from build123d import *

# Parameters (mm, degrees)
F1_DEPTH       = 25.4
F2_SIZE        = 20.32
F5_R           = 6.35
F6_DEPTH       = 25.4
F6_DEPTH_BACK  = 25.4
F7_R           = 3.81
F8_DEPTH       = 46.228
F8_DEPTH_BACK  = 55.88
F9_R           = 6.35
F10_DEPTH      = 25.4
F10_DEPTH_BACK = 25.4
F11_R          = 3.81
F12_DEPTH      = 41.402
F12_DEPTH_BACK = 45.212
F13_R          = 5.08


# Not quite as in the source:
# - a feature of the source that left no trace in its solid (it failed there, or was rolled back) is left out


with BuildPart() as f1:
    # F0 (on Front) → F1 (new body)
    with BuildSketch(Plane.XZ):
        Polygon((0, 57.15), (-25.0849546432, 41.8481773181), (-25.0849546432, -41.8481773181), (0, -57.15), (25.0849546432, -41.8481773181), (25.0849546432, 41.8481773181), align=None)
    extrude(amount=F1_DEPTH)

    # F2
    f2_edges = [f1.edges().sort_by_distance(p)[0] for p in [
        (-12.542477, -25.4, 49.499089),
        (12.542477, -25.4, 49.499089),
    ]]
    chamfer(f2_edges, length=F2_SIZE)

    # F5 (on Right) → F6 (join, two sides)
    with BuildSketch(Plane.YZ) as f6_sk:
        with Locations((0, -29.1547831148)):
            Circle(F5_R)
    extrude(amount=-F6_DEPTH)
    extrude(f6_sk.sketch, amount=F6_DEPTH_BACK)

    # F7 (on Right) → F8 (cut, two sides)
    with BuildSketch(Plane.YZ) as f8_sk:
        with Locations((0, -29.1547831148)):
            Circle(F7_R)
    extrude(amount=-F8_DEPTH, mode=Mode.SUBTRACT)
    extrude(f8_sk.sketch, amount=F8_DEPTH_BACK, mode=Mode.SUBTRACT)

    # F9 (on Right) → F10 (join, two sides)
    with BuildSketch(Plane.YZ) as f10_sk:
        with Locations((0, 22.8599980474)):
            Circle(F9_R)
    extrude(amount=F10_DEPTH)
    extrude(f10_sk.sketch, amount=-F10_DEPTH_BACK)

    # F11 (on Right) → F12 (cut, two sides)
    with BuildSketch(Plane.YZ) as f12_sk:
        with Locations((0, 22.8599980474)):
            Circle(F11_R)
    extrude(amount=-F12_DEPTH, mode=Mode.SUBTRACT)
    extrude(f12_sk.sketch, amount=F12_DEPTH_BACK, mode=Mode.SUBTRACT)

    # F13
    f13_edges = [f1.edges().sort_by_distance(p)[0] for p in [
        (-25.084955, -25.4, -11.901086),
        (-12.542477, -25.4, 25.696917),
        (-12.542477, -25.4, -49.499089),
        (12.542477, -25.4, 25.696917),
        (12.542477, -25.4, -49.499089),
        (25.084955, -25.4, -11.901086),
    ]]
    fillet(f13_edges, radius=F13_R)


solid = f1.part
The model under review builds one solid part; all positions refer to its coordinate system, in mm. A direction names the side the tool comes from. Give positions to 0.01 mm unless a question says otherwise; leave off trailing zeros. Write each loop counter-clockwise with the first axis right and the second up, starting at its lowest first coordinate (ties: lowest second). Pieces come first, ordered by that corner, then holes. Notation, with made-up numbers: M -28.5,86.25 L -10.5,86.25 A19 ccw -10.5,94.25 Z; hole C 49.5,-8.75 d3. An arc over 180 degrees is marked long. One line per question, with ' | ' between items. Start each with the question number.
Item 1: For pin 1 (4.5 mm diameter, centred on y = 0, z = 22.86, fed in from +X); pin 2 (19.5 mm diameter, centred on x = 10.5, z = -2, fed in from +Y); pin 3 (6 mm diameter, centred on y = -12, z = 6.5, fed in from +X); pin 4 (1 mm diameter, centred on y = -15.5, z = -19.5, fed in from -X), all flat-tipped, find the tip position at first contact; note any pin that passes through.
Item 2: For faces 1 (the flat face through (0, 0, 40)), 2 (the flat face through (0, 0, -44)), 3 (the flat face through (25.085, -10, -1)), list the 3-axis set-ups (+Z, -Z, +X, -X, +Y, -Y) from which the entire face can be reached by the end or side of a thin tool; tool diameter is ignored.
Item 3: We need section A-A on z = -26.5. Write out the cut boundary in (x, y), plus the area to 3 significant figures.
Item 4: We need section B-B on y = -14. Write out the cut boundary in (x, z), plus the area to 3 significant figures.
Item 5: We need section C-C on z = 14.5. Write out the cut boundary in (x, y).
Item 6: We need section D-D on x = 3.5. Give the number of separate pieces and of enclosed holes in the cut face, plus the area to 3 significant figures.
Item 7: Wall thickness on line 1 (Z direction, x = -3, y = 0.5); line 2 (Y direction, x = -1.5, z = 14.5); line 3 (X direction, y = -10.5, z = -19): over which ranges is each line inside the solid? List them lowest first. Write a range as from..to.
Results found:
1) pin 1: passes through | pin 2: stops at y = 0 | pin 3: stops at x = 25.08 | pin 4: stops at x = -25.08
2) face 1: +Z, +X, -X, +Y | face 2: -Z, +X, -X, +Y | face 3: +X, -Y
3) outline: M -25.4,-5.77 L -25.08,-5.77 L -25.08,-20.32 A5.08 ccw -20,-25.4 L 20,-25.4 A5.08 ccw 25.08,-20.32 L 25.08,-5.77 L 25.4,-5.77 L 25.4,-2.73 L -25.4,-2.73 Z; M -25.4,2.73 L 25.4,2.73 L 25.4,5.77 L -25.4,5.77 Z | area: 1,280 mm2
4) outline: M -25.08,-41.85 L 0,-57.15 L 25.08,-41.85 L 25.08,31.4 L 0,46.7 L -25.08,31.4 Z | area: 4,440 mm2
5) outline: M -25.08,-20.32 A5.08 ccw -20,-25.4 L 20,-25.4 A5.08 ccw 25.08,-20.32 L 25.08,0 L -25.08,0 Z
6) separate pieces: 1 | enclosed holes: 2 | area: 2,580 mm2
7) line 1: z = -35.49..-32.93, -25.38..-22.82, 16.53..19.08, 26.64..29.19 | line 2: y = -25.4..0 | line 3: x = -25.08..25.08
